Can you work these out from the model? Positions are in its coordinate system, mm. Face numbers are marked on the shaded views. Coordinates: 2 decimals unless noted, no trailing zeros.
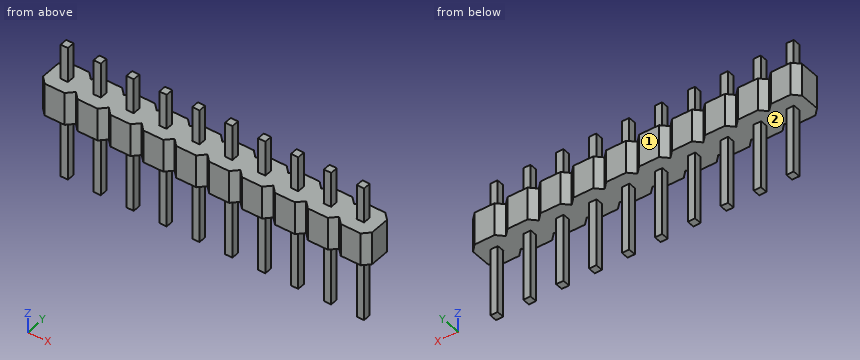
```python
from build123d import *

# Parameters (mm, degrees)
SKETCH1_W                = 0.58
SKETCH1_H                = 0.58
BOSS_EXTRUDE1_DEPTH      = 2.54
SKETCH2_W                = 0.5591264
SKETCH2_H                = 0.575944702
BOSS_EXTRUDE2_DEPTH      = 5.25
BOSS_EXTRUDE2_DEPTH_BACK = 5.25


with BuildPart() as part:
    # Sketch1 → Boss-Extrude1 (new body)
    with BuildSketch(Plane.XY):
        Polygon((-37.946397324, 14.279123168), (-37.446397324, 14.779123168), (-35.906397324, 14.779123168), (-35.406397324, 14.279123168), (-34.906397324, 14.779123168), (-33.366397324, 14.779123168), (-32.866397324, 14.279123168), (-32.366397324, 14.779123168), (-30.826397324, 14.779123168), (-30.326397324, 14.279123168), (-29.826397324, 14.779123168), (-28.286397324, 14.779123168), (-27.786397324, 14.279123168), (-27.286397324, 14.779123168), (-25.746397324, 14.779123168), (-25.246397324, 14.279123168), (-24.746397324, 14.779123168), (-23.206397324, 14.779123168), (-22.706397324, 14.279123168), (-22.206397324, 14.779123168), (-20.666397324, 14.779123168), (-20.166397324, 14.279123168), (-19.666397324, 14.779123168), (-18.126397324, 14.779123168), (-17.626397324, 14.279123168), (-17.126397324, 14.779123168), (-15.586397324, 14.779123168), (-15.086397324, 14.279123168), (-14.586397324, 14.779123168), (-13.046397324, 14.779123168), (-12.546397324, 14.279123168), (-12.546397324, 12.739123168), (-13.046397324, 12.239123168), (-14.586397324, 12.239123168), (-15.086397324, 12.739123168), (-15.586397324, 12.239123168), (-17.126397324, 12.239123168), (-17.626397324, 12.739123168), (-18.126397324, 12.239123168), (-19.666397324, 12.239123168), (-20.166397324, 12.739123168), (-20.666397324, 12.239123168), (-22.206397324, 12.239123168), (-22.706397324, 12.739123168), (-23.206397324, 12.239123168), (-24.746397324, 12.239123168), (-25.246397324, 12.739123168), (-25.746397324, 12.239123168), (-27.286397324, 12.239123168), (-27.786397324, 12.739123168), (-28.286397324, 12.239123168), (-29.826397324, 12.239123168), (-30.326397324, 12.739123168), (-30.826397324, 12.239123168), (-32.366397324, 12.239123168), (-32.866397324, 12.739123168), (-33.366397324, 12.239123168), (-34.906397324, 12.239123168), (-35.406397324, 12.739123168), (-35.906397324, 12.239123168), (-37.446397324, 12.239123168), (-37.946397324, 12.739123168), align=None)
        with Locations((-16.356397324, 13.509123168)):
            Rectangle(SKETCH1_W, SKETCH1_H, mode=Mode.SUBTRACT)
        with Locations((-13.816397324, 13.509123168)):
            Rectangle(SKETCH1_W, SKETCH1_H, mode=Mode.SUBTRACT)
        with Locations((-18.896397324, 13.509123168)):
            Rectangle(SKETCH1_W, SKETCH1_H, mode=Mode.SUBTRACT)
        with Locations((-21.436397324, 13.509123168)):
            Rectangle(SKETCH1_W, SKETCH1_H, mode=Mode.SUBTRACT)
        with Locations((-23.976397324, 13.509123168)):
            Rectangle(SKETCH1_W, SKETCH1_H, mode=Mode.SUBTRACT)
        with Locations((-26.516397324, 13.509123168)):
            Rectangle(SKETCH1_W, SKETCH1_H, mode=Mode.SUBTRACT)
        with Locations((-29.056397324, 13.509123168)):
            Rectangle(SKETCH1_W, SKETCH1_H, mode=Mode.SUBTRACT)
        with Locations((-31.596397324, 13.509123168)):
            Rectangle(SKETCH1_W, SKETCH1_H, mode=Mode.SUBTRACT)
        with Locations((-34.136397324, 13.509123168)):
            Rectangle(SKETCH1_W, SKETCH1_H, mode=Mode.SUBTRACT)
        with Locations((-36.676397324, 13.509123168)):
            Rectangle(SKETCH1_W, SKETCH1_H, mode=Mode.SUBTRACT)
    extrude(amount=BOSS_EXTRUDE1_DEPTH)

    # Sketch2 → Boss-Extrude2 (add, two sides)
    with BuildSketch(Plane.XY) as boss_extrude2_sk:
        with Locations((-16.345960524, 13.511150817)):
            Rectangle(SKETCH2_W, SKETCH2_H)
        with Locations((-13.805960524, 13.511150817)):
            Rectangle(SKETCH2_W, SKETCH2_H)
        with Locations((-18.885960524, 13.511150817)):
            Rectangle(SKETCH2_W, SKETCH2_H)
        with Locations((-21.425960524, 13.511150817)):
            Rectangle(SKETCH2_W, SKETCH2_H)
        with Locations((-23.965960524, 13.511150817)):
            Rectangle(SKETCH2_W, SKETCH2_H)
        with Locations((-26.505960524, 13.511150817)):
            Rectangle(SKETCH2_W, SKETCH2_H)
        with Locations((-29.045960524, 13.511150817)):
            Rectangle(SKETCH2_W, SKETCH2_H)
        with Locations((-31.585960524, 13.511150817)):
            Rectangle(SKETCH2_W, SKETCH2_H)
        with Locations((-34.125960524, 13.511150817)):
            Rectangle(SKETCH2_W, SKETCH2_H)
        with Locations((-36.665960524, 13.511150817)):
            Rectangle(SKETCH2_W, SKETCH2_H)
    extrude(amount=BOSS_EXTRUDE2_DEPTH)
    extrude(boss_extrude2_sk.sketch, amount=-BOSS_EXTRUDE2_DEPTH_BACK)


solid = part.part
```
Item 1: I need wall thicknesses on line 1 along Y through (x, z) = (-16.5, -3); line 2 along Z through (x, y) = (-17.5, 13.5); line 3 along Y through (x, z) = (-32.5, 0.75). Which ranges of each line are inside material? Lowest first, please.
Results are:
line 1: y = 13.22 to 13.8
line 2: z = 0 to 2.54
line 3: y = 12.37 to 14.65
Item 2: Suppose I cut it at A-A, the plane z = 1.5. Count the separate pieces of the cut face and the enclosed holes in it, plus the area to 3 significant figures.
Results are:
separate pieces: 1
enclosed holes: 10
area: 59.4 mm2
Item 3: We'd pull the mould along X, two halves only. Please class the marked faces 1 and 2: +X half, -X half, draft (parallel to the pull), parting line (faces both ways), or undercut.
Results are:
face 1: draft
face 2: undercut
Item 4: I'm going to push flat-ended pins straight in: P1, Ø1, axis at x = -19.5, z = -3.5, coming from the -Y side; P2, Ø5, axis at x = -21, z = 3.5, coming from the -Y side. Where does each tip first touch, or does it pass through?
Results are:
P1: stops at y = 13.22
P2: stops at y = 12.24
